Check sheet for the modelled part. Datum: model origin and axes. Units: mm. Face numbers are marked on the shaded views. A direction names the side the tool comes from. Coordinates: 2 decimals unless noted, no trailing zeros. Loops run counter-clockwise (first coordinate to the right, second up) from the corner with the lowest first, then second, coordinate; pieces in that order, holes last. Notation, with made-up numbers: (50, -38) - (61, -38) arc R31 ccw to (61, -14) - close; hole circle Ø7 at (17, 30.25). An arc over 180 degrees is marked (long way). Use a Markdown table: item, result. Add a question column.
1) Draft check along X on the marked faces 3, 4, 5 and 6. Enter one of: pulls with the +X half, pulls with the -X half, needs draft (parallel to the pull), parting line crosses it, or undercut.
2) Sectioned sample at B-B, the plane z = -3.5. Enter the section's corners in (x, y).
3) Sectioned sample at A-A, the plane y = 14.25. Enter the section's corners in (x, z).
4) Sectioned sample at C-C, the plane x = 1. Enter the section's corners in (y, z).
5) Tool access check on the marked faces 1 and 2. Record the directions out of +Z, -Z, +X, -X, +Y, -Y that give a thin tool (end or side, any length) a straight path to the whole face; none if there is none.
6) Thickness scan on line 1 (Z direction, x = 7, y = 5.75); line 2 (X direction, y = 21.5, z = -0.5); line 3 (X direction, y = 26.75, z = -9). Record the ranges inside material, lowest first.
from build123d import *

# Parameters (mm, degrees)
F0_W     = 30
F0_H     = 15
F1_DEPTH = 1.2
F0_W_2   = 32.4
F0_H_2   = 17.4
F2_DEPTH = 29.2
F3_R     = 2


with BuildPart() as f1:
    # F0 (on Front) → F1 (new body)
    with BuildSketch(Plane.XZ):
        with Locations((0.849122, -7.366886)):
            Rectangle(F0_W, F0_H)
    extrude(amount=-F1_DEPTH)

    # F0 (on Front) → F2 (join)
    with BuildSketch(Plane.XZ):
        with Locations((0.849122, -7.366886)):
            Rectangle(F0_W_2, F0_H_2)
        with Locations((0.849122, -7.366886)):
            Rectangle(F0_W, F0_H, mode=Mode.SUBTRACT)
    extrude(amount=-F2_DEPTH)

    # F3
    f3_edges = [f1.edges().sort_by_distance(p)[0] for p in [
        (17.049122, 14.6, 1.333114),
        (0.849122, 0, 1.333114),
        (0.849122, 0, -16.066886),
        (17.049122, 0, -7.366886),
        (17.049122, 14.6, -16.066886),
        (-15.350878, 0, -7.366886),
        (-15.350878, 14.6, 1.333114),
        (-15.350878, 14.6, -16.066886),
    ]]
    fillet(f3_edges, radius=F3_R)


solid = f1.part
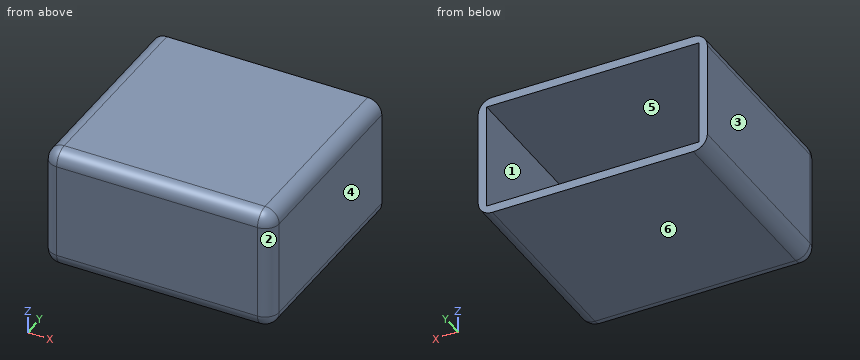
Solved:
| question | item | result |
|---|---|---|
| 1 | face 3 | pulls with the -X half |
| 1 | face 4 | pulls with the +X half |
| 1 | face 5 | undercut |
| 1 | face 6 | needs draft |
| 2 | outline | (-15.35, 2) arc R2 ccw to (-13.35, 0) - (15.05, 0) arc R2 ccw to (17.05, 2) - (17.05, 29.2) - (15.85, 29.2) - (15.85, 1.2) - (-14.15, 1.2) - (-14.15, 29.2) - (-15.35, 29.2) - close |
| 3 | outline | (-15.35, -14.07) arc R2 ccw to (-13.35, -16.07) - (15.05, -16.07) arc R2 ccw to (17.05, -14.07) - (17.05, -0.67) arc R2 ccw to (15.05, 1.33) - (-13.35, 1.33) arc R2 ccw to (-15.35, -0.67) - close; hole (-14.15, -14.87) - (15.85, -14.87) - (15.85, 0.13) - (-14.15, 0.13) - close |
| 4 | outline | (0, -14.07) arc R2 ccw to (2, -16.07) - (29.2, -16.07) - (29.2, -14.87) - (1.2, -14.87) - (1.2, 0.13) - (29.2, 0.13) - (29.2, 1.33) - (2, 1.33) arc R2 ccw to (0, -0.67) - close |
| 5 | face 1 | +Y |
| 5 | face 2 | +Z, -Z, +X, -Y |
| 6 | line 1 | z = -16.07 to -14.87, 0.13 to 1.33 |
| 6 | line 2 | x = -15.34 to -14.15, 15.85 to 17.04 |
| 6 | line 3 | x = -15.35 to -14.15, 15.85 to 17.05 |
